from build123d import *

# Parameters (mm, degrees)
SKETCH1_W           = 310
SKETCH1_H           = 250
BOSS_EXTRUDE1_DEPTH = 1
SKETCH2_OUTSIDE_W   = 391.65
SKETCH2_OUTSIDE_H   = 331.65
CUT_EXTRUDE1_DEPTH  = 200.125588511
SKETCH3_R           = 15.25
SKETCH3_R_2         = 8.25
SKETCH3_R_3         = 11.25
SKETCH3_R_4         = 1.6
SKETCH3_R_5         = 1
CUT_EXTRUDE2_DEPTH  = 200.125588511
SKETCH4_R           = 8.25
CUT_EXTRUDE3_DEPTH  = 200.125588511
SKETCH5_R           = 3
CUT_EXTRUDE4_DEPTH  = 200.125588511


with BuildPart() as part:
    # Sketch1 → Boss-Extrude1 (new body)
    with BuildSketch(Plane(origin=(0, 0, 0), x_dir=(0, 1, 0), z_dir=(0, 0, 1))):
        Rectangle(SKETCH1_W, SKETCH1_H)
    extrude(amount=BOSS_EXTRUDE1_DEPTH)

    # Sketch2 outside → Cut-Extrude1 (cut, through all)
    with BuildSketch(Plane(origin=(0, 0, 1), x_dir=(0, -1, 0), z_dir=(0, 0, 1))):
        Rectangle(SKETCH2_OUTSIDE_W, SKETCH2_OUTSIDE_H)
        Polygon((-155, -14.047727215), (155, -124.233933248), (155, 125), (-110.452272785, 125), (-155, 80.452272785), align=None, mode=Mode.SUBTRACT)
    extrude(amount=-CUT_EXTRUDE1_DEPTH, mode=Mode.SUBTRACT)

    # Sketch3 → Cut-Extrude2 (cut, through all)
    with BuildSketch(Plane(origin=(0, 0, 1), x_dir=(0, -1, 0), z_dir=(0, 0, 1))):
        with Locations(Location((-105, 60, 0), (0, 0, 90))):
            Circle(SKETCH3_R)
        with Locations(Location((-45, 60, 0), (0, 0, 90))):
            Circle(SKETCH3_R_2)
        with Locations(Location((15, 60, 0), (0, 0, 90))):
            Circle(SKETCH3_R_3)
        with Locations(Location((-105, 35.251262658, 0), (0, 0, 90))):
            Circle(SKETCH3_R_4)
        with Locations(Location((-129.748737342, 60, 0), (0, 0, 90))):
            Circle(SKETCH3_R_4)
        with Locations(Location((-105, 84.748737342, 0), (0, 0, 90))):
            Circle(SKETCH3_R_4)
        with Locations(Location((-80.251262658, 60, 0), (0, 0, 90))):
            Circle(SKETCH3_R_4)
        with Locations(Location((15, 74, 0), (0, 0, 90))):
            Circle(SKETCH3_R_5)
        with Locations(Location((15, 46, 0), (0, 0, 90))):
            Circle(SKETCH3_R_5)
    extrude(amount=-CUT_EXTRUDE2_DEPTH, mode=Mode.SUBTRACT)

    # Sketch4 → Cut-Extrude3 (cut, through all)
    with BuildSketch(Plane(origin=(0, 0, 1), x_dir=(0, -1, 0), z_dir=(0, 0, 1))):
        with Locations(Location((125, -59.616966624, 0), (0, 0, 90))):
            Circle(SKETCH4_R)
        with Locations(Location((125, -29.616966624, 0), (0, 0, 90))):
            Circle(SKETCH4_R)
        with Locations(Location((125, 0.383033376, 0), (0, 0, 90))):
            Circle(SKETCH4_R)
        with Locations(Location((125, 30.383033376, 0), (0, 0, 90))):
            Circle(SKETCH4_R)
        with Locations(Location((125, 60.383033376, 0), (0, 0, 90))):
            Circle(SKETCH4_R)
    extrude(amount=-CUT_EXTRUDE3_DEPTH, mode=Mode.SUBTRACT)

    # Sketch5 → Cut-Extrude4 (cut, through all)
    with BuildSketch(Plane(origin=(0, 0, 1), x_dir=(0, -1, 0), z_dir=(0, 0, 1))):
        with Locations(Location((145, -110.066636279, 0), (0, 0, 90))):
            Circle(SKETCH5_R)
        with Locations(Location((-145, -6.989217732, 0), (0, 0, 90))):
            Circle(SKETCH5_R)
        with Locations(Location((-145, 76.310137162, 0), (0, 0, 90))):
            Circle(SKETCH5_R)
        with Locations(Location((145, 115, 0), (0, 0, 90))):
            Circle(SKETCH5_R)
        with Locations(Location((-106.310137162, 115, 0), (0, 0, 90))):
            Circle(SKETCH5_R)
    extrude(amount=-CUT_EXTRUDE4_DEPTH, mode=Mode.SUBTRACT)


solid = part.part
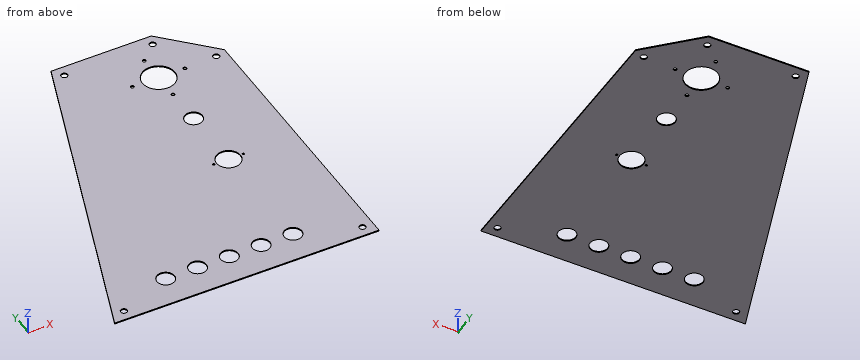
Part model, mm, in its own coordinate system. Give positions to 0.01 mm unless a question says otherwise; leave off trailing zeros. Order: outer loops, then holes, each group sorted by start corner. A loop starts at its lowest first (then second) coordinate and runs counter-clockwise, first axis right, second up. Notation, with made-up numbers: (16.25, 40.25) - (38.25, 40.25) arc R20 cw to (38.25, 67.25) - close; hole circle Ø3 at (82.5, 88.5). An arc over 180 degrees is marked (long way). One line per question, with ' | ' between items.
1. Band-saw the part on B-B on z = 0.55. Give the number of separate pieces and of enclosed holes in the cut face, then the cut area to 3 significant figures.
Filled in:
separate pieces: 1 | enclosed holes: 19 | area: 56,600 mm²
2. Drill centre lines: probe 1 along X at (y, z) = (-145, 0.2); probe 2 along X at (y, z) = (145, 0.3); probe 3 along Y at (x, z) = (36, 0.1). Where is each one in solid material? Low to high.
Filled in:
probe 1: -120.68 to -113.07, -107.07 to 112, 118 to 125 | probe 2: -17.6 to -9.99, -3.99 to 73.31, 79.31 to 90.45 | probe 3: -155 to -131.04, -118.96 to 103.59, 106.41 to 155
3. Drop a flat-ended pin along its axis: P1, Ø8, axis at x = 115, y = -145, coming from the -Z side. Give the stop position or say it passes through.
Filled in:
P1: z = 0
4. Band-saw the part on A-A on y = -125. List the corners of the cut face in (x, z), then the cut area to 3 significant figures.
Filled in:
outline: (-113.57, 0) - (-67.87, 0) - (-67.87, 1) - (-113.57, 1) - close; (-51.37, 0) - (-37.87, 0) - (-37.87, 1) - (-51.37, 1) - close; (-21.37, 0) - (-7.87, 0) - (-7.87, 1) - (-21.37, 1) - close; (8.63, 0) - (22.13, 0) - (22.13, 1) - (8.63, 1) - close; (38.63, 0) - (52.13, 0) - (52.13, 1) - (38.63, 1) - close; (68.63, 0) - (125, 0) - (125, 1) - (68.63, 1) - close | area: 156 mm²
5. Band-saw the part on C-C on y = -73.5. List the corners of the cut face in (x, z).
Filled in:
outline: (-95.27, 0) - (125, 0) - (125, 1) - (-95.27, 1) - close
6. Band-saw the part on D-D on x = -73.5. List the corners of the cut face in (y, z).
Filled in:
outline: (-155, 0) - (-12.26, 0) - (-12.26, 1) - (-155, 1) - close
